Geometry check sheet. Reference: the model listing, model coordinates, mm. Round coordinates to 2 decimals unless told otherwise and drop trailing zeros. Write each loop counter-clockwise with the first axis right and the second up, starting at its lowest first coordinate (ties: lowest second). Pieces come first, ordered by that corner, then holes. Notation, with made-up numbers: (30.25, 1) -> (53.25, 1) arc R25 cw to (53.25, 38) -> close; hole circle Ø2 at (57, -29.75). An arc over 180 degrees is marked (long way). One line per question, with ' | ' between items.
```python
from build123d import *

# Parameters (mm, degrees)
F0_W           = 100
F0_H           = 125
F0_R           = 7.3677826157
F1_DEPTH       = 1.5
F3_D           = 2
F3_CSINK_D     = 4
F3_CSINK_ANGLE = 90


# Not quite as in the source:
# - a feature names something its author has since deleted; it is built from what else it names


with BuildPart() as f1:
    # F0 (on Front) → F1 (new body)
    with BuildSketch(Plane.XZ):
        Rectangle(F0_W, F0_H)
        with BuildLine():
            Line((-34.9434472264, -7.1068441343), (-8.9434472264, -7.1068441343))
            ThreePointArc((-8.9434472264, -7.1068441343), (-3.9936997581, -9.157096666), (-1.9434472264, -14.1068441343))
            Line((-1.9434472264, -14.1068441343), (-1.9434472264, -45.5))
            ThreePointArc((-1.9434472264, -45.5), (-3.9936997581, -50.4497474683), (-8.9434472264, -52.5))
            Line((-8.9434472264, -52.5), (-34.9434472264, -52.5))
            ThreePointArc((-34.9434472264, -52.5), (-39.8931946947, -50.4497474683), (-41.9434472264, -45.5))
            Line((-41.9434472264, -45.5), (-41.9434472264, -14.1068441343))
            ThreePointArc((-41.9434472264, -14.1068441343), (-39.8931946947, -9.157096666), (-34.9434472264, -7.1068441343))
        make_face(mode=Mode.SUBTRACT)
        with BuildLine():
            ThreePointArc((41.9434472264, -45.5), (39.8931946947, -50.4497474683), (34.9434472264, -52.5))
            Line((34.9434472264, -52.5), (8.9434472264, -52.5))
            ThreePointArc((8.9434472264, -52.5), (3.9936997581, -50.4497474683), (1.9434472264, -45.5))
            Line((1.9434472264, -45.5), (1.9434472264, -14.1068441343))
            ThreePointArc((1.9434472264, -14.1068441343), (3.9936997581, -9.157096666), (8.9434472264, -7.1068441343))
            Line((8.9434472264, -7.1068441343), (34.9434472264, -7.1068441343))
            ThreePointArc((34.9434472264, -7.1068441343), (39.8931946947, -9.157096666), (41.9434472264, -14.1068441343))
            Line((41.9434472264, -14.1068441343), (41.9434472264, -45.5))
        make_face(mode=Mode.SUBTRACT)
        with BuildLine():
            ThreePointArc((-1.9434472264, 14.1068441343), (-3.9936997581, 9.157096666), (-8.9434472264, 7.1068441343))
            Line((-8.9434472264, 7.1068441343), (-34.9434472264, 7.1068441343))
            ThreePointArc((-34.9434472264, 7.1068441343), (-39.8931946947, 9.157096666), (-41.9434472264, 14.1068441343))
            Line((-41.9434472264, 14.1068441343), (-41.9434472264, 45.5))
            ThreePointArc((-41.9434472264, 45.5), (-39.8931946947, 50.4497474683), (-34.9434472264, 52.5))
            Line((-34.9434472264, 52.5), (-8.9434472264, 52.5))
            ThreePointArc((-8.9434472264, 52.5), (-3.9936997581, 50.4497474683), (-1.9434472264, 45.5))
            Line((-1.9434472264, 45.5), (-1.9434472264, 14.1068441343))
        make_face(mode=Mode.SUBTRACT)
        Circle(F0_R, mode=Mode.SUBTRACT)
        with BuildLine():
            ThreePointArc((8.9434472264, 7.1068441343), (3.9936997581, 9.157096666), (1.9434472264, 14.1068441343))
            Line((1.9434472264, 14.1068441343), (1.9434472264, 45.5))
            ThreePointArc((1.9434472264, 45.5), (3.9936997581, 50.4497474683), (8.9434472264, 52.5))
            Line((8.9434472264, 52.5), (34.9434472264, 52.5))
            ThreePointArc((34.9434472264, 52.5), (39.8931946947, 50.4497474683), (41.9434472264, 45.5))
            Line((41.9434472264, 45.5), (41.9434472264, 14.1068441343))
            ThreePointArc((41.9434472264, 14.1068441343), (39.8931946947, 9.157096666), (34.9434472264, 7.1068441343))
            Line((34.9434472264, 7.1068441343), (8.9434472264, 7.1068441343))
        make_face(mode=Mode.SUBTRACT)
    extrude(amount=F1_DEPTH)

    # F3 (through all)
    with Locations(Plane.XZ.offset(1.5)):
        with Locations((-43.5, -59.5), (43.5, -59.5), (43.5, 59.5), (-43.5, 59.5)):
            CounterSinkHole(F3_D / 2, F3_CSINK_D / 2, counter_sink_angle=F3_CSINK_ANGLE)


solid = f1.part
```
(1) Sectioned sample at B-B on x = -32.5. Record the cut outline in (y, z), then the cut area to 3 significant figures.
Resolved:
outline: (-1.5, -62.5) -> (0, -62.5) -> (0, -52.5) -> (-1.5, -52.5) -> close; (-1.5, -7.11) -> (0, -7.11) -> (0, 7.11) -> (-1.5, 7.11) -> close; (-1.5, 52.5) -> (0, 52.5) -> (0, 62.5) -> (-1.5, 62.5) -> close | area: 51.3 mm2
(2) Sectioned sample at C-C on x = 0. Record the cut outline in (y, z), then the cut area to 3 significant figures.
Resolved:
outline: (-1.5, -62.5) -> (0, -62.5) -> (0, -7.37) -> (-1.5, -7.37) -> close; (-1.5, 7.37) -> (0, 7.37) -> (0, 62.5) -> (-1.5, 62.5) -> close | area: 165 mm2
(3) Material ranges on line 1 (X direction, y = -0.15, z = 59.5); line 2 (Z direction, x = 43.5, y = -0.2); line 3 (Z direction, x = -32, y = -0.2), recorded low to high.
Resolved:
line 1: x = -50 to -44.5, -42.5 to 42.5, 44.5 to 50 | line 2: z = -62.5 to -60.5, -58.5 to 58.5, 60.5 to 62.5 | line 3: z = -62.5 to -52.5, -7.11 to 7.11, 52.5 to 62.5
(4) Go/stop test with a flat-tipped pin: pin 1 (1.2 mm diameter, centred on x = -43.5, z = 59.5, fed in from -Y). Record where the tip stops, or that it passes through.
Resolved:
pin 1: passes through
(5) Draft check along Z on faces 1 (the flat face through (-12, 0, 1)), 2 (the cylindrical face through (39.947, -0.74, 9.212)). Enter one of: +Z half, -Z half, draft (parallel to the pull), parting line (faces both ways), or undercut.
Resolved:
face 1: draft | face 2: undercut
(6) Sectioned sample at A-A on z = -18.5. Record the cut outline in (x, y), then the cut area to 3 significant figures.
Resolved:
outline: (-50, -1.5) -> (-41.94, -1.5) -> (-41.94, 0) -> (-50, 0) -> close; (-1.94, -1.5) -> (1.94, -1.5) -> (1.94, 0) -> (-1.94, 0) -> close; (41.94, -1.5) -> (50, -1.5) -> (50, 0) -> (41.94, 0) -> close | area: 30.0 mm2
(7) Sectioned sample at D-D on y = -0.8. Count the separate pieces of the cut face and the enclosed holes in it, then the cut area to 3 significant figures.
Resolved:
separate pieces: 1 | enclosed holes: 9 | area: 5,210 mm2
